Source: CAD feature listing. Evaluate the final solid. Frame: model axes, mm. Face numbers are marked on the shaded views. A direction names the side the tool comes from. Give positions to 0.01 mm unless a question says otherwise; leave off trailing zeros. Loops run counter-clockwise (first coordinate to the right, second up) from the corner with the lowest first, then second, coordinate; pieces in that order, holes last. Notation, with made-up numbers: (-35.5, 10.5) -> (6.5, 10.5) arc R6 cw to (6.5, 15.5) -> close; hole circle Ø10 at (10, 21.5). An arc over 180 degrees is marked (long way). Return JSON: item names as keys, results as strings. Group by question number.
(1) Cut plane D-D on z = -6.25. Return loops of the section in (x, y).
(2) Cut plane C-C on y = 3.25. Return loops of the section in (x, z) (3 decimals), then the cut area to 3 significant figures.
(3) Cut plane A-A on y = 0. Return loops of the section in (x, z) (3 decimals).
(4) Cut plane B-B on x = -1. Return loops of the section in (y, z) (3 decimals), then the cut area to 3 significant figures.
(5) Access query for the marked faces 1 and 2. Directions: +Z, -Z, +X, -X, +Y, -Y. A direction counts if a zero-diameter tool reaches every point of the face in a straight line with its end or side. Return the directions, or none.
(6) Pin query (flat end, axial travel): pin 1 (2.5 mm diameter, centred on y = 0, z = -5.6, fed in from -X); pin 2 (3 mm diameter, centred on y = -2.5, z = 4.5, fed in from -X); pin 3 (1.5 mm diameter, centred on y = 2.5, z = 7.5, fed in from +X). Return the tip coordinate at first contact, or that it passes through.
(7) Ray query, line 1 (Z direction, x = 0.5, y = 0) (3 decimals); line 2 (Z direction, x = 2.75, y = 0.5) (3 decimals); line 3 (Z direction, x = 0.75, y = 4.5). Return the intervals inside material, ascending. Write a range as from..to.
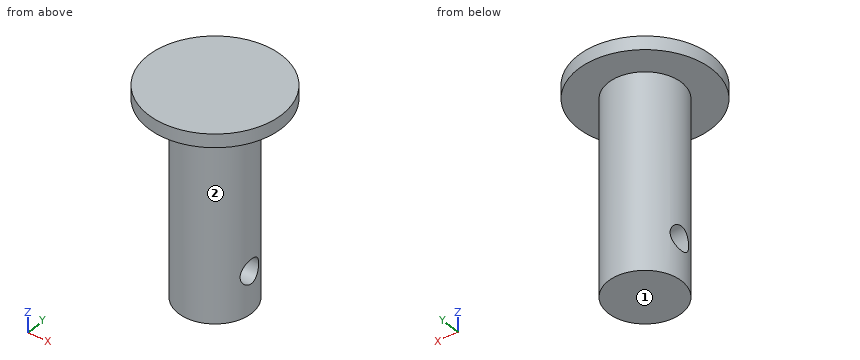
```python
from build123d import *

# Parameters (mm, degrees)
F0_R     = 3.466188
F1_DEPTH = 9.525
F2_R     = 6.327639
F3_DEPTH = 0.635
F4_R     = 1.138516
F5_DEPTH = 12.7


with BuildPart() as f1:
    # F0 (on Top) → F1 (new body, symmetric)
    with BuildSketch(Plane.XY):
        Circle(F0_R)
    extrude(amount=F1_DEPTH, both=True)

    # F2 (on face) → F3 (join, symmetric)
    with BuildSketch(Plane.XY.offset(9.525)):
        Circle(F2_R)
    extrude(amount=F3_DEPTH, both=True)

    # F4 (on Right) → F5 (cut, symmetric)
    with BuildSketch(Plane.YZ):
        with Locations((0, -5.598677)):
            Circle(F4_R)
    extrude(amount=F5_DEPTH, both=True, mode=Mode.SUBTRACT)


solid = f1.part
```
Answers:
{
 "1": {"outline": "(-3.34, -0.93) arc R3.47 ccw to (3.34, -0.93) -> close; (-3.34, 0.93) -> (3.34, 0.93) arc R3.47 ccw to start"},
 "2": {"outline": "(-5.429, 8.89) -> (-1.205, 8.89) -> (-1.205, -9.525) -> (1.205, -9.525) -> (1.205, 8.89) -> (5.429, 8.89) -> (5.429, 10.16) -> (-5.429, 10.16) -> close", "area": "58.2 mm²"},
 "3": {"outline": "(-6.328, 8.89) -> (-3.466, 8.89) -> (-3.466, -4.46) -> (3.466, -4.46) -> (3.466, 8.89) -> (6.328, 8.89) -> (6.328, 10.16) -> (-6.328, 10.16) -> close; (-3.466, -9.525) -> (3.466, -9.525) -> (3.466, -6.737) -> (-3.466, -6.737) -> close"},
 "4": {"outline": "(-6.248, 8.89) -> (-3.319, 8.89) -> (-3.319, -9.525) -> (3.319, -9.525) -> (3.319, 8.89) -> (6.248, 8.89) -> (6.248, 10.16) -> (-6.248, 10.16) -> close; hole circle Ø2.277 at (0, -5.599)", "area": "134 mm²"},
 "5": {"face 1": "-Z, +X, -X, +Y, -Y", "face 2": "-Z"},
 "6": {"pin 1": "x = -3.47", "pin 2": "x = -3.32", "pin 3": "x = 2.99"},
 "7": {"line 1": "-9.525..-6.737, -4.46..10.16", "line 2": "-9.525..-6.622, -4.576..10.16", "line 3": "8.89..10.16"}
}
